Model file for the job. Use its own axes, mm. Face numbers are marked on the shaded views. A direction names the side the tool comes from. Coordinates: 2 decimals unless noted, no trailing zeros. Loops run counter-clockwise (first coordinate to the right, second up) from the corner with the lowest first, then second, coordinate; pieces in that order, holes last.
Autodesk Inventor part; units mm, degrees
ref_plane "YZ Plane" through (0, 0, 0) normal (1, 0, 0) x (0, 1, 0)
ref_plane "XZ Plane" through (0, 0, 0) normal (0, 1, 0) x (-1, 0, 0)
ref_plane "XY Plane" through (0, 0, 0) normal (0, 0, 1) x (1, 0, 0)
sketch "Sketch1" plane through (0, 0, 0) normal (0, 0, 1) x (1, 0, 0)
  line L0 (0, 0) -> (79.43, 0)
  line L1 (79.43, 0) -> (79.43, -10)
  line L2 (79.43, -10) -> (0, -10)
  line L3 (0, -10) -> (0, 0)
  line L4 (79.43, 0) -> (43.93, 0)
  line L5 (43.93, 0) -> (43.93, 14.475)
  line L6 (43.93, 14.475) -> (79.43, 14.475)
  line L7 (79.43, 14.475) -> (79.43, 0)
  line L8 (3.2, 0) -> (6.4, 0) construction
  line L9 (6.4, 0) -> (6.4, -10) construction
  line L10 (6.4, -10) -> (3.2, -10) construction
  line L11 (3.2, -10) -> (3.2, 0) construction
  line L12 (4.8, 0) -> (4.8, -10) construction
  line L13 (55.93, 14.475) -> (55.93, -10) construction
  line L14 (70.93, 14.475) -> (70.93, -10) construction
  line L15 (53.43, 14.475) -> (58.43, 14.475) construction
  line L16 (58.43, 14.475) -> (58.43, -10) construction
  line L17 (58.43, -10) -> (53.43, -10) construction
  line L18 (53.43, -10) -> (53.43, 14.475) construction
  line L19 (68.43, 14.475) -> (73.43, 14.475) construction
  line L20 (73.43, 14.475) -> (73.43, -10) construction
  line L21 (73.43, -10) -> (68.43, -10) construction
  line L22 (68.43, -10) -> (68.43, 14.475) construction
  dimension "d0" = 14.475
  dimension "d3" = 3.2
  dimension "d4" = 3.2
  dimension "d6" = 39.13
  dimension "d34" = 10
  dimension "d35" = 5
  dimension "d36" = 5
  dimension "d37" = 2.5
  dimension "d38" = 2.5
  dimension "d39" = 12
  dimension "d40" = 10
  dimension "d41" = 6
extrude "Extrusion1" add sketch "Sketch1" along normal blind 12
sketch "Sketch2" plane through (43.93, 14.475, 0) normal (0, 1, 0) x (1, 0, 0)
  line L0 (35.5, 0) -> (0, 0)
  line L1 (0, 0) -> (0, -12)
  line L2 (35.5, -12) -> (0, -12)
  line L3 (35.5, 0) -> (35.5, -12)
  line L4 (0, 0) -> (0, -12)
  line L5 (0, 0) -> (-43.93, 0)
  line L6 (-43.93, 0) -> (-43.93, -12)
  line L7 (0, -12) -> (-43.93, -12)
  circle A0 centre (-39.13, -6) radius 1.6
  circle A1 centre (29, -6) radius 2.5
  circle A2 centre (14, -6) radius 2.5
  dimension "d15" = 3.2
  dimension "d16" = 5
  dimension "d17" = 5
  dimension "d22" = 12
  dimension "d23" = 6
  dimension "d24" = 6
  dimension "d26" = 3.2
  dimension "d42" = 14
  dimension "d43" = 10
extrude "Extrusion2" cut sketch "Sketch2" against normal up to surface (24.475 mm away) contours A0 | A1 | A2
fillet "Fillet1" radius 3 2 edges at (43.93, 14.475, 6) (43.93, 0, 6)
sketch "Sketch3" plane through (0, 0, 12) normal (0, 1, 0) x (1, 0, 0)
  line L0 (40.93, 12) -> (40.93, 0)
  line L1 (40.93, 12) -> (0, 12)
  line L2 (0, 12) -> (0, 0)
  line L3 (40.93, 0) -> (0, 0)
  circle A0 centre (4.8, 6) radius 1.6
  circle A1 centre (4.8, 6) radius 2.5
  circle A2 centre (4.8, 6) radius 1.6
  circle A3 centre (4.8, 6) radius 1.6
  dimension "d31" = 5
extrude "Extrusion3" add sketch "Sketch3" along normal blind 1.5 contours A1
sketch "Sketch4" plane through (0, 0, 12) normal (0, 1, 0) x (1, 0, 0)
  line L0 (43.93, 0) -> (43.93, 12)
  line L1 (43.93, 12) -> (43.93, 0)
  circle A0 centre (4.8, 6) radius 2.5
  line L2 (40.93, 12) -> (40.93, 0)
  line L3 (40.93, 12) -> (0, 12)
  line L4 (0, 12) -> (0, 0)
  line L5 (40.93, 0) -> (0, 0)
  line L6 (43.93, 12) -> (43.93, 0)
  line L7 (43.93, 0) -> (43.93, 12)
  line L8 (0, 12) -> (79.43, 12)
  line L9 (15.63, 12) -> (35.63, 12)
  line L10 (35.63, 12) -> (35.63, 0)
  line L11 (35.63, 0) -> (15.63, 0)
  line L12 (15.63, 0) -> (15.63, 12)
  dimension "d44" = 8.3
  dimension "d45" = 20
extrude "Extrusion4" add sketch "Sketch4" along normal blind 2.5 contours L10 L5 L12 L3
equation "\"d37\" = 0.5 * d35"
equation "\"d38\" = 0.5 * d36"
properties part number "BottomWheelHolder"
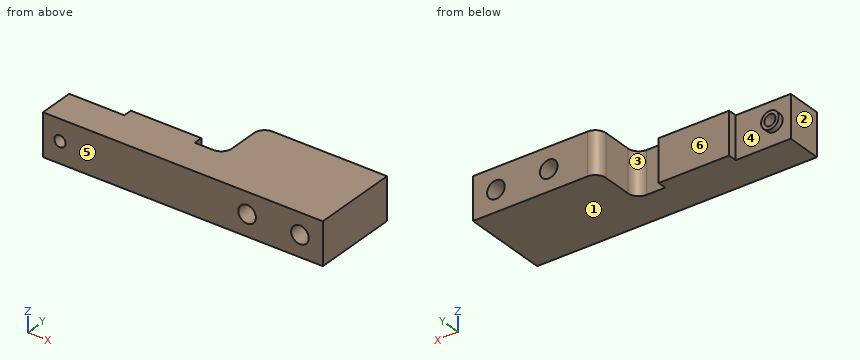
Q1. Drill centre lines: line 1 (X direction, y = 9.5, z = 6.25); line 2 (X direction, y = -1.75, z = 6); line 3 (Z direction, x = 72.93, y = 2.5). Where is each one in solid material? Low to high.
Answers:
line 1: x = 43.93 to 55.44, 60.42 to 70.44, 75.42 to 79.43
line 2: x = 0 to 3.2, 6.4 to 55.43, 60.43 to 70.43, 75.43 to 79.43
line 3: z = 0 to 3.5, 8.5 to 12
Q2. Which spindle directions (+Z, -Z, +X, -X, +Y, -Y) get a long thin tool onto all of the face, cutting with end or side? Do the marked faces 5 and 6. Say none if no direction does.
Answers:
face 5: +Z, -Z, +X, -X, -Y
face 6: +Z, -Z, -X, +Y
Q3. Slice it at A-A (x = 4.8). List the corners of the cut face in (y, z).
Answers:
outline: (-10, 0) - (0, 0) - (0, 3.5) - (1.5, 3.5) - (1.5, 4.4) - (-10, 4.4) - close; (-10, 7.6) - (1.5, 7.6) - (1.5, 8.5) - (0, 8.5) - (0, 12) - (-10, 12) - close
Q4. Flat gauge pins, fed straight in: P1, Ø2, axis at x = 26, y = 4, coming from the +Z side; P2, Ø1.6, axis at x = 38, z = 6, coming from the +Y side; P3, Ø5.5, axis at x = 4.5, z = 6.5, coming from the +Y side; P4, Ø0.8, axis at y = 1, z = 8.5, coming from the -X side. Where does each tip first touch, or does it go through?
Answers:
P1: passes through
P2: stops at y = 0
P3: stops at y = 1.5
P4: stops at x = 3.44
Q5. Mould opens along X. For the marked faces 1, 2, 3 and 4 say: +X half, -X half, draft (parallel to the pull), parting line (faces both ways), or undercut.
Answers:
face 1: draft
face 2: -X half
face 3: undercut
face 4: undercut
Q6. Slice it at B-B (z = 6). List the corners of the cut face in (x, y) (3 decimals).
Answers:
outline: (0, -10) - (3.2, -10) - (3.2, 1.5) - (2.3, 1.5) - (2.3, 0) - (0, 0) - close; (6.4, -10) - (55.43, -10) - (55.43, 14.475) - (46.93, 14.475) arc R3 ccw to (43.93, 11.475) - (43.93, 3) arc R3 cw to (40.93, 0) - (35.63, 0) - (35.63, 2.5) - (15.63, 2.5) - (15.63, 0) - (7.3, 0) - (7.3, 1.5) - (6.4, 1.5) - close; (60.43, -10) - (70.43, -10) - (70.43, 14.475) - (60.43, 14.475) - close; (75.43, -10) - (79.43, -10) - (79.43, 14.475) - (75.43, 14.475) - close
Q7. Slice it at D-D (x = 57.93). List the corners of the cut face in (y, z) (3 decimals).
Answers:
outline: (-10, 0) - (14.475, 0) - (14.475, 3.5) - (-10, 3.5) - close; (-10, 8.5) - (14.475, 8.5) - (14.475, 12) - (-10, 12) - close
Q8. Slice it at C-C (y = -5.75). List the corners of the cut face in (x, z).
Answers:
outline: (0, 0) - (79.43, 0) - (79.43, 12) - (0, 12) - close; hole circle Ø3.2 at (4.8, 6); hole circle Ø5 at (57.93, 6); hole circle Ø5 at (72.93, 6)
